Can you work these out from the model? Positions are in its coordinate system, mm. A direction names the side the tool comes from. Give positions to 0.01 mm unless a question says otherwise; leave off trailing zeros. Write each loop counter-clockwise with the first axis right and the second up, starting at its lowest first coordinate (ties: lowest second). Pieces come first, ordered by that corner, then holes.
1. Suppose I cut it at A-A (x = -4). Please give me the cut outline in (y, z), and give its area (3 significant figures).
2. Thinking about a two-plate mould opening in Y: for faces 1 (the flat face through (0, -7.5, 1)), 2 (the cylindrical face through (0, 0, 1)), 3 (the flat face through (0, 7.5, 1)), 4 (the flat face through (-5, -5, 1)), which applies, pulls with the +Y half, pulls with the -Y half, needs draft (parallel to the pull), parting line crosses it, or undercut?
3. Suppose I cut it at C-C (y = 0). Please give me the cut outline in (x, z).
4. Suppose I cut it at B-B (z = 1.8). Please give me the cut outline in (x, y), and give its area (3 significant figures).
5. Suppose I cut it at D-D (y = -1.75). Please give me the cut outline in (x, z).
6. On a 3-axis mill with a long thin cutter (end or side, diameter ignored), from which of +Z, -Z, +X, -X, +Y, -Y can I reach the whole of each face in a straight line? I mean faces 5 (the flat face through (-5, 5, 1)), 6 (the flat face through (-4, 2.5, 1)). Say none if no direction works.
7. If I drill on probe 1 along Y at (x, z) = (-3.25, 1.2); probe 2 along Y at (x, z) = (-1, 1.5); probe 3 along X at (y, z) = (0.5, 0.25), over which ranges is the centre line in solid material (lowest first)?
```python
from build123d import *

# Parameters (mm, degrees)
BOSS_EXTRUDE1_DEPTH = 2


with BuildPart() as part:
    # Sketch1 → Boss-Extrude1 (new body)
    with BuildSketch(Plane.XY):
        with BuildLine():
            Line((-5, 2.5), (-5, 7.5))
            Line((-5, 7.5), (5, 7.5))
            Line((5, 7.5), (5, -7.5))
            Line((5, -7.5), (-5, -7.5))
            Line((-5, -7.5), (-5, -2.5))
            Line((-5, -2.5), (-2.5, -2.5))
            ThreePointArc((-2.5, -2.5), (0, 0), (-2.5, 2.5))
            Line((-2.5, 2.5), (-5, 2.5))
        make_face()
    extrude(amount=BOSS_EXTRUDE1_DEPTH)


solid = part.part
```
Checks:
1. outline: (-7.5, 0) - (-2.5, 0) - (-2.5, 2) - (-7.5, 2) - close; (2.5, 0) - (7.5, 0) - (7.5, 2) - (2.5, 2) - close
1. area: 20.0 mm2
2. face 1: pulls with the -Y half
2. face 2: undercut
2. face 3: pulls with the +Y half
2. face 4: needs draft
3. outline: (0, 0) - (5, 0) - (5, 2) - (0, 2) - close
4. outline: (-5, -7.5) - (5, -7.5) - (5, 7.5) - (-5, 7.5) - (-5, 2.5) - (-2.5, 2.5) arc R2.5 cw to (-2.5, -2.5) - (-5, -2.5) - close
4. area: 128 mm2
5. outline: (-0.71, 0) - (5, 0) - (5, 2) - (-0.71, 2) - close
6. face 5: +Z, -Z, -X, +Y, -Y
6. face 6: +Z, -Z, -X
7. probe 1: y = -7.5 to -2.5, 2.5 to 7.5
7. probe 2: y = -7.5 to -2, 2 to 7.5
7. probe 3: x = -0.05 to 5
